Source: CAD feature listing. Evaluate the final solid. Frame: model axes, mm. A direction names the side the tool comes from. Round coordinates to 2 decimals unless told otherwise and drop trailing zeros. Loops run counter-clockwise (first coordinate to the right, second up) from the corner with the lowest first, then second, coordinate; pieces in that order, holes last. Notation, with made-up numbers: (29, 78.25) -> (86, 78.25) arc R23 ccw to (86, 117.25) -> close; hole circle Ø1 at (5, -16). An arc over 180 degrees is marked (long way). Return JSON: item names as keys, results as strings. Group by question number.
```python
from build123d import *

# Parameters (mm, degrees)
F1_DEPTH    = 25.4
F2_T2_ANGLE = 136.8806858284
F2_T4_ANGLE = 136.8806858284
F2_T6_ANGLE = 136.8806858284
F2_T8_ANGLE = 136.8806858285
F3_R        = 1.3857299945
F4_DEPTH    = 2.3622
F5_R        = 2.5973758292
F5_R_2      = 1.5258073578
F6_DEPTH    = 2.54
F7_R        = 0.6147751451
F8_DEPTH    = 7.6708


# Not quite as in the source:
# - a fillet or chamfer that OpenCascade refuses, or shapes differently, is made with other operations: its cross-section is extruded or revolved along the edge and cut away or added
# - a feature names something its author has since deleted; it is built from what else it names


with BuildPart() as f1:
    # F0 (on Front) → F1 (new body)
    with BuildSketch(Plane.XZ):
        with BuildLine():
            Line((9.9314, -5.7745984882), (9.9314, 5.7745984882))
            ThreePointArc((9.9314, 5.7745984882), (9.3786903902, 6.6346710713), (8.7517057092, 7.4422))
            Line((8.7517057092, 7.4422), (-8.7517057092, 7.4422))
            ThreePointArc((-8.7517057092, 7.4422), (-9.3786903902, 6.6346710713), (-9.9314, 5.7745984882))
            Line((-9.9314, 5.7745984882), (-9.9314, -5.7745984882))
            ThreePointArc((-9.9314, -5.7745984882), (-9.3786903902, -6.6346710713), (-8.7517057092, -7.4422))
            Line((-8.7517057092, -7.4422), (8.7517057092, -7.4422))
            ThreePointArc((8.7517057092, -7.4422), (9.3786903902, -6.6346710713), (9.9314, -5.7745984882))
        make_face()
    extrude(amount=F1_DEPTH)

    # F2: fillet of radius 5.08 on 4 edges, made by hand

    # F2_s1 → F2_t2 (revolve, cut)
    with BuildSketch(Plane(origin=(0, 0, 0), x_dir=(0, 1, 0), z_dir=(0.9714801037, 0, -0.2371210832))):
        with BuildLine():
            ThreePointArc((-20.32, 11.4881980162), (-23.9121024484, 10.0003004647), (-25.4, 6.4081980162))
            Line((-25.4, 6.4081980162), (-25.4, 11.4881980162))
            Line((-25.4, 11.4881980162), (-20.32, 11.4881980162))
        make_face()
    revolve(axis=Axis((0, -25.4, 0), (0, -1, 0)), revolution_arc=F2_T2_ANGLE, mode=Mode.SUBTRACT)

    # F2_s3 → F2_t4 (revolve, cut)
    with BuildSketch(Plane(origin=(0, 0, 0), x_dir=(0, 1, 0), z_dir=(-0.5470373523, 0, -0.837108198))):
        with BuildLine():
            ThreePointArc((-20.32, 11.4881980162), (-23.9121024484, 10.0003004647), (-25.4, 6.4081980162))
            Line((-25.4, 6.4081980162), (-25.4, 11.4881980162))
            Line((-25.4, 11.4881980162), (-20.32, 11.4881980162))
        make_face()
    revolve(axis=Axis((0, -25.4, 0), (0, -1, 0)), revolution_arc=F2_T4_ANGLE, mode=Mode.SUBTRACT)

    # F2_s5 → F2_t6 (revolve, cut)
    with BuildSketch(Plane(origin=(0, 0, 0), x_dir=(0, 1, 0), z_dir=(0.5470373523, 0, 0.837108198))):
        with BuildLine():
            ThreePointArc((-20.32, 11.4881980162), (-23.9121024484, 10.0003004647), (-25.4, 6.4081980162))
            Line((-25.4, 6.4081980162), (-25.4, 11.4881980162))
            Line((-25.4, 11.4881980162), (-20.32, 11.4881980162))
        make_face()
    revolve(axis=Axis((0, -25.4, 0), (0, -1, 0)), revolution_arc=F2_T6_ANGLE, mode=Mode.SUBTRACT)

    # F2_s7 → F2_t8 (revolve, cut)
    with BuildSketch(Plane(origin=(0, 0, 0), x_dir=(0, 1, 0), z_dir=(-0.9714801037, 0, 0.2371210832))):
        with BuildLine():
            ThreePointArc((-20.32, 11.4881980162), (-23.9121024484, 10.0003004647), (-25.4, 6.4081980162))
            Line((-25.4, 6.4081980162), (-25.4, 11.4881980162))
            Line((-25.4, 11.4881980162), (-20.32, 11.4881980162))
        make_face()
    revolve(axis=Axis((0, -25.4, 0), (0, -1, 0)), revolution_arc=F2_T8_ANGLE, mode=Mode.SUBTRACT)

    # F3 (on face) → F4 (join)
    with BuildSketch(Plane.XZ.offset(25.4)):
        with BuildLine():
            ThreePointArc((1.5195188547, 6.2254368734), (-5.231499759, 3.7008663967), (-5.364355094, -3.5055236756))
            ThreePointArc((-5.364355094, -3.5055236756), (-2.3548191815, -5.9598513771), (1.5195188547, -6.2254368734))
            ThreePointArc((1.5195188547, -6.2254368734), (3.7008663967, -5.231499759), (5.364355094, -3.5055236756))
            ThreePointArc((5.364355094, -3.5055236756), (5.9598513771, 2.3548191815), (1.5195188547, 6.2254368734))
        make_face()
        Circle(F3_R, mode=Mode.SUBTRACT)
    extrude(amount=F4_DEPTH)

    # F5 (on face) → F6 (join)
    with BuildSketch(Plane.XZ):
        Circle(F5_R)
        Circle(F5_R_2, mode=Mode.SUBTRACT)
    extrude(amount=-F6_DEPTH)

    # F7 (on Front) → F8 (join)
    with BuildSketch(Plane.XZ):
        Circle(F7_R)
    extrude(amount=-F8_DEPTH)


solid = f1.part
```
(1) Set-up query: faces 1 (the face through (-0.563, 1.252, -2.536)), 2 (the face through (0, 7.671, 0)). Return all of +Z, -Z, +X, -X, +Y, -Y with unobstructed straight access to the full face (end or side cutting, diameter ignored); none if empty.
(2) Mould query, pull axis Z, two halves, no side actions, for faces 3 (the face through (-9.37, -10.02, 6.65)), 4 (the face through (-0.3, -26.565, -1.353)), 5 (the face through (0, -27.762, 2)), 6 (the face through (0, -25.4, 0)). Classes: released by +Z, released by -Z, zero draft, split by the parting line, or undercut.
(3) Pin query (flat end, axial travel): pin 1 (7.5 mm diameter, centred on x = 3, z = 3, fed in from +Y); pin 2 (4 mm diameter, centred on x = 0, z = -5, fed in from +Y); pin 3 (0.8 mm diameter, centred on x = -0.5, z = 0, fed in from -Y). Return the tip coordinate at first contact, or that it passes through.
(4) Cut plane B-B (z = 0). Return loops of the section in (x, y), and give its area (3 significant figures).
(5) Cut plane C-C (y = -23). Return loops of the section in (x, z), and give its area (3 significant figures).
(6) Ray query, line 1 (Z direction, x = 0, y = 0.6); line 2 (Z direction, x = 0, y = -26.2); line 3 (Y direction, x = -1.75, z = 1.25). Return the intervals inside material, ascending.
(7) Cut plane D-D (y = 3.5). Return loops of the section in (x, z), and give its area (3 significant figures).
(8) Cut plane A-A (x = 0). Return loops of the section in (y, z).
Answers follow:
{
 "1": {"face 1": "+Y", "face 2": "+Z, -Z, +X, -X, +Y"},
 "2": {"face 3": "released by +Z", "face 4": "undercut", "face 5": "zero draft", "face 6": "undercut"},
 "3": {"pin 1": "y = 7.67", "pin 2": "y = 0", "pin 3": "y = -25.4"},
 "4": {"outline": "(-9.93, -23.98) arc R5.08 ccw to (-6.41, -25.4) -> (-6.41, -27.76) -> (-1.39, -27.76) -> (-1.39, -25.4) -> (1.39, -25.4) -> (1.39, -27.76) -> (6.41, -27.76) -> (6.41, -25.4) arc R5.08 ccw to (9.93, -23.98) -> (9.93, 0) -> (2.6, 0) -> (2.6, 2.54) -> (1.53, 2.54) -> (1.53, 0) -> (0.61, 0) -> (0.61, 7.67) -> (-0.61, 7.67) -> (-0.61, 0) -> (-1.53, 0) -> (-1.53, 2.54) -> (-2.6, 2.54) -> (-2.6, 0) -> (-9.93, 0) -> close", "area": "540 mm^2"},
 "5": {"outline": "(-9.93, -4.05) arc R10.72 ccw to (-7.72, -7.44) -> (7.72, -7.44) arc R10.72 ccw to (9.93, -4.05) -> (9.93, 4.05) arc R10.72 ccw to (7.72, 7.44) -> (-7.72, 7.44) arc R10.72 ccw to (-9.93, 4.05) -> close", "area": "283 mm^2"},
 "6": {"line 1": "-2.6 to -1.53, -0.61 to 0.61, 1.53 to 2.6", "line 2": "-6.41 to -1.39, 1.39 to 6.41", "line 3": "-27.76 to 2.54"},
 "7": {"outline": "circle Ø1.23 at (0, 0)", "area": "1.19 mm^2"},
 "8": {"outline": "(-27.76, -6.41) -> (-25.4, -6.41) arc R5.08 ccw to (-25.29, -7.44) -> (0, -7.44) -> (0, -2.6) -> (2.54, -2.6) -> (2.54, -1.53) -> (0, -1.53) -> (0, -0.61) -> (7.67, -0.61) -> (7.67, 0.61) -> (0, 0.61) -> (0, 1.53) -> (2.54, 1.53) -> (2.54, 2.6) -> (0, 2.6) -> (0, 7.44) -> (-25.29, 7.44) arc R5.08 ccw to (-25.4, 6.41) -> (-27.76, 6.41) -> (-27.76, 1.39) -> (-25.4, 1.39) -> (-25.4, -1.39) -> (-27.76, -1.39) -> close"}
}
